Build history of the part. All positions in model axes, mm. A direction names the side the tool comes from. Give positions to 0.01 mm unless a question says otherwise; leave off trailing zeros. Write each loop counter-clockwise with the first axis right and the second up, starting at its lowest first coordinate (ties: lowest second). Pieces come first, ordered by that corner, then holes.
from build123d import *


with BuildPart() as part:
    # Sketch1 → Revolve1 (revolve)
    with BuildSketch(Plane.XY):
        Polygon((-120, 0), (120, 0), (120, 44.5), (-100, 44.5), (-100, 54.5), (-120, 54.5), align=None)
    revolve(axis=Axis((-120, 0, 0), (1, 0, 0)))

    # Sketch2 → Cut-Revolve2 (revolve, cut)
    with BuildSketch(Plane.XY):
        with BuildLine():
            Line((66.48120035, 0), (266.48120035, 0))
            ThreePointArc((266.48120035, 0), (197.846476125, 79.188575606), (109.710437686, 22.5))
            Line((109.710437686, 22.5), (66.48120035, 22.5))
            Line((66.48120035, 22.5), (66.48120035, 0))
        make_face()
    revolve(axis=Axis((66.48120035, 0, 0), (1, 0, 0)), mode=Mode.SUBTRACT)


solid = part.part
1. Drill centre lines: line 1 along Z through (x, y) = (86, 0); line 2 along X through (y, z) = (-15, -17); line 3 along X through (y, z) = (21, 49.5). Where is each one in solid material? Low to high.
2. Mould opens along Y. For faces 3 (the face through (66.481, 0, 0)), 4 (the face through (-110.14, -43.25, -33.16)), 5 (the face through (-100, 45, 0)) say: pulls with the +Y half, pulls with the -Y half, needs draft (parallel to the pull), parting line crosses it, or undercut.
3. Saw through at B-B on y = -32. Give the cut face in (x, z).
4. Drop flat-ended pins along their axis: pin 1 (13.5 mm diameter, centred on y = -8, z = 8, fed in from +X); pin 2 (12 mm diameter, centred on x = 45.5, y = -34.5, fed in from +Z); pin 3 (8 mm diameter, centred on x = -56, z = 6.5, fed in from +Y). Give the stop position or say it passes through.
5. 3-axis set-ups, long thin cutter, end or side, ignore diameter. For faces 1 (the face through (-120, -1, 1)), 2 (the face through (8.46, -32.798, 30.075)): which of +Z, -Z, +X, -X, +Y, -Y reach the whole face in a straight line?
6. Saw through at A-A on z = 0. Give the cut face in (x, y), plus the area to 3 significant figures.
7. Saw through at D-D on x = 79. Give the cut face in (y, z).
8. Saw through at C-C on x = -78. Give the cut face in (y, z).
Outcome:
1. line 1: z = -44.5 to -22.5, 22.5 to 44.5
1. line 2: x = -120 to 109.76
1. line 3: x = -120 to -100
2. face 3: undercut
2. face 4: parting line crosses it
2. face 5: needs draft
3. outline: (-120, -44.12) - (-100, -44.12) - (-100, -30.92) - (120, -30.92) arc R73.32 cw to (120, 30.92) - (-100, 30.92) - (-100, 44.12) - (-120, 44.12) - close
4. pin 1: stops at x = 66.48
4. pin 2: stops at z = 34.18
4. pin 3: stops at y = 44.43
5. face 1: +Z, -Z, -X, +Y, -Y
5. face 2: +X
6. outline: (-120, -54.5) - (-100, -54.5) - (-100, -44.5) - (120, -44.5) arc R80 cw to (109.71, -22.5) - (66.48, -22.5) - (66.48, 22.5) - (109.71, 22.5) arc R80 cw to (120, 44.5) - (-100, 44.5) - (-100, 54.5) - (-120, 54.5) - close
6. area: 19,100 mm2
7. outline: circle Ø89 at (0, 0); hole circle Ø45 at (0, 0)
8. outline: circle Ø89 at (0, 0)
